Autodesk Inventor part; units mm, degrees
ref_plane "Work Plane1" through (0, 15, 0) normal (0, 1, 0) x (1, 0, 0)
ref_plane "Work Plane2" through (30.5, 0, 0) normal (1, 0, 0) x (0, 1, 0)
ref_plane "Work Plane6" through (0, 0, 2) normal (0, 0, 1) x (1, 0, 0)
sketch "Sketch1" plane through (0, 0, 0) normal (0, 1, 0) x (-1, 0, 0)
  circle A0 centre (0, 0) radius 26.5
  circle A1 centre (0, 0) radius 30.5
  dimension "d0" = 53
  dimension "d1" = 4
extrude "Extrusion1" add sketch "Sketch1" along normal blind 22
extrude "Extrusion2" add sketch "Sketch1" against normal blind 4 contours A0 | A1
ref_plane "Work Plane1" through (0, 15, 0) normal (0, 1, 0) x (1, 0, 0)
ref_plane "Work Plane2" through (30.5, 0, 0) normal (1, 0, 0) x (0, 1, 0)
sketch "Sketch3" plane through (30.5, 0, 0) normal (1, 0, 0) x (0, 1, 0)
  line L0 (14, -18.4883) -> (14, 18.4883)
  line L1 (16, 18.4883) -> (16, -18.4883)
  line L2 (16, 21.067) -> (16, 18.4883)
  line L3 (14, 18.4883) -> (14, 21.067)
  line L4 (16, 21.067) -> (16, -21.067)
  line L5 (16, 21.067) -> (16, 18.4883)
  line L6 (16, 18.4883) -> (16, -18.4883)
  line L7 (16, -18.4883) -> (16, -21.067)
  line L8 (14, -21.067) -> (14, -18.4883)
  line L9 (23, 32.2933) -> (-6, 32.2933)
  line L10 (-6, 32.2933) -> (-6, -38.454)
  line L11 (-6, -38.454) -> (23, -38.454)
  line L12 (23, -38.454) -> (23, 32.2933)
  line L13 (23, 24.5) -> (-6, 24.5)
  line L14 (23, -24.5) -> (-6.5731, -24.5)
  line L15 (-4, 30.5) -> (22, 30.5)
  line L16 (-4, -30.5) -> (22, -30.5)
  point P0 (0, 0)
  point P1 (-6, -24.5)
  dimension "d11" = 7
  dimension "d12" = 20
  dimension "d31" = 6
  dimension "d32" = 6
extrude "Extrusion4" cut sketch "Sketch3" against normal through all contours L12 L13 L10 L9 | L12 L11 L10 L14
sketch "Sketch4" plane through (0, 15, 0) normal (0, 1, 0) x (1, 0, 0)
  point P0 (0, 0)
ref_plane "Work Plane6" through (0, 0, 2) normal (0, 0, 1) x (1, 0, 0)
ref_plane "Work Plane5" through (0, 0, 30.5) normal (0, 0, 1) x (1, 0, 0)
sketch "Sketch6" plane through (0, 0, 2) normal (0, 0, 1) x (1, 0, 0)
  point P0 (0, 0)
sketch "Sketch7" plane through (0, 0, 2) normal (0, 0, 1) x (1, 0, 0)
  line L0 (-30.5, -4) -> (30.5, -4)
  line L1 (0, -4) -> (0, -71)
  circle A0 centre (0, -71) radius 57
  circle A1 centre (0, -71) radius 59.5
  circle A2 centre (0, -12.7932) radius 2.25
  circle A3 centre (-12.0008, -14) radius 2.25
  line L2 (4.6794, -4) -> (4.6794, -18.4597)
  line L3 (4.6794, -18.4597) -> (-15.0336, -19.4972)
  line L4 (-15.0336, -19.4972) -> (-17.1884, -4)
  point P0 (0, 0)
  dimension "d24" = 67
  dimension "d25" = 114
  dimension "d26" = 119
  dimension "d27" = 4.5
  dimension "d28" = 4.5
extrude "Extrusion6" add sketch "Sketch7" along normal mid plane 16 contours L0 L1 A2 A1 A3 L4 | L0 L2 A1 A2 L1 | A1 A3 A0 L4 | A0 A3 A2 L1 L3 L4 | L2 A0 A2 A1 | A2 A0 A3 A1 | L2 L3 L1 A2 A0
sketch "Sketch8" plane through (-18.1659, -4, 24.5) normal (0, 0, 1) x (1, 0, 0)
  line L0 (28.2654, 26) -> (36.3318, 26)
  line L1 (36.3318, 0) -> (0, 0)
  line L2 (36.3318, 26) -> (28.2654, 26)
  line L3 (28.2654, 26) -> (28.2654, 0)
  line L4 (28.2654, 0) -> (36.3318, 0)
  line L5 (36.3318, 0) -> (36.3318, 26)
  line L6 (28.2654, 4) -> (28.2654, 26)
  line L7 (0, 0) -> (0, 26)
  line L8 (36.3318, 0) -> (0, 0)
  line L9 (0, 0) -> (0, 4)
  line L10 (0, 4) -> (36.3318, 4)
  line L11 (36.3318, 4) -> (36.3318, 0)
  line L12 (8.0664, 26) -> (8.0664, 4)
  line L13 (0, 0) -> (8.0664, 0)
  line L14 (8.0664, 0) -> (8.0664, 26)
  line L15 (8.0664, 26) -> (0, 26)
  line L16 (0, 26) -> (0, 0)
  point P0 (18.1659, 4)
  dimension "d33" = 0
extrude "Extrusion7" add sketch "Sketch8" along normal blind 2
sketch "Sketch9" plane through (-18.1659, -4, 26.5) normal (0, 0, 1) x (1, 0, 0)
  line L0 (0, 0) -> (36.3318, 0)
  line L1 (8.0664, 26) -> (0, 26)
  line L2 (36.3318, 0) -> (0, 0)
  line L3 (0, 0) -> (0, 26)
  line L4 (0, 26) -> (36.3318, 26)
  line L5 (36.3318, 26) -> (36.3318, 0)
  line L6 (20.1659, 9) -> (16.1659, 9)
  line L7 (16.1659, 9) -> (16.1659, 26)
  line L8 (16.1659, 26) -> (20.1659, 26)
  line L9 (20.1659, 26) -> (20.1659, 9)
  line L10 (28.2654, 4) -> (8.0664, 4)
  point P0 (18.1659, 4)
  point P1 (18.1659, 4)
  point P2 (18.1659, 9)
  point P3 (18.1659, 4)
  dimension "d36" = 4
  dimension "d37" = 0
  dimension "d38" = 5
  dimension "d39" = 0
extrude "Extrusion8" add sketch "Sketch9" along normal blind 1 contours L3 L1 L4 L7 L6 L9 L5 L0
mirror "Mirror1" about plane through (0, 0, 0) normal (0, 0, 1) of "Extrusion8", "Extrusion7"
sketch "Sketch10" plane through (0, 22, 0) normal (0, 1, 0) x (1, 0, 0)
  circle A0 centre (0, 0) radius 28.75
  line L0 (10.0995, -24.5) -> (10.0995, -26.5)
  line L1 (10.0995, -26.5) -> (11.74, -26.5)
  line L2 (10.0995, -26.5) -> (11.74, -26.5) construction
  line L3 (11.74, -26.5) -> (-11.1496, -26.5)
  line L4 (27.6145, -8) -> (-27.6145, -8)
  point P0 (0, -8)
  point P1 (11.1496, -26.5)
  dimension "d42" = 57.5
  dimension "d43" = 0
  dimension "d44" = 8
extrude "Extrusion9" cut sketch "Sketch10" against normal up to surface (22 mm away) contours L4 A0 L1 L3
chamfer "Chamfer1" distance 2.25 angle 45 2 edges at (-25.2636, 11, 8) (25.2636, 11, 8)
mirror "Mirror2" about plane through (0, 0, 0) normal (0, 0, 1) of "Extrusion9"
chamfer "Chamfer2" distance 2.25 angle 45 2 edges at (-25.2636, 11, -8) (25.2636, 11, -8)
ref_plane "Work Plane7" through (4.6794, -4, 1) normal (0.1736, -0.9848, 0) x (0, 0, -1)
sketch "Sketch11" plane through (4.6794, -4, 1) normal (0.1736, -0.9848, 0) x (0, 0, -1)
  line L0 (-26.5, -22.4982) -> (-26.5, 13.2817)
  line L1 (28.5, -22.4982) -> (28.5, 13.2817)
  line L2 (7, -2.5109) -> (-9, -2.5109)
  line L3 (-9, 0) -> (7, 0)
  circle A0 centre (1, 0) radius 2.15
  point P0 (1, -3.9137)
  dimension "d54" = 4.3
  dimension "d55" = 27.5
extrude "Extrusion10" cut sketch "Sketch11" along normal through all both and the other way through all
ref_plane "Work Plane3" through (30.5, 0, 0) normal (1, 0, 0) x (0, 1, 0)
sketch "Sketch5" plane through (2, 0, 0) normal (1, 0, 0) x (0, 1, 0)
  line L0 (-4, 30.5) -> (-4, -30.5)
  line L1 (-4, 0) -> (-71, 0)
  circle A0 centre (-71, 0) radius 57
  circle A1 centre (-71, 0) radius 59.5
  circle A2 centre (-12.675, 0) radius 1.5
  circle A3 centre (-14.6323, 14.7617) radius 1.5
  line L2 (-4, -4.4838) -> (-16.1323, -4.4838)
  line L3 (-16.1323, -4.4838) -> (-19.3598, 18.592)
  line L4 (-19.3598, 18.592) -> (-4, 18.9349)
  point P0 (0, 0)
  dimension "d16" = 67
  dimension "d17" = 114
  dimension "d18" = 119
  dimension "d19" = 3
  dimension "d20" = 3
properties part number "BigLif2"
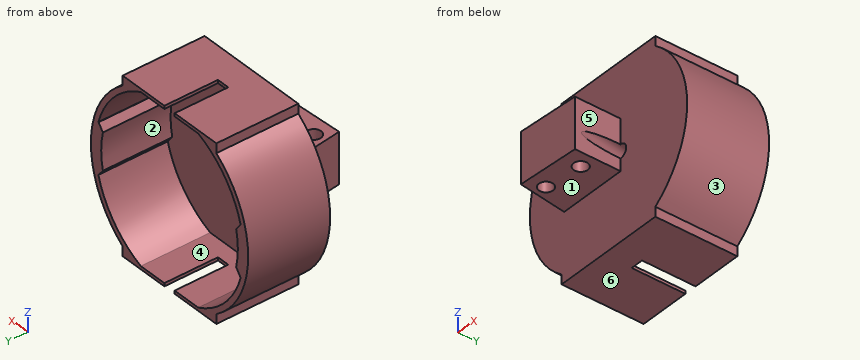
CAD build for the part. Positions are in the model's coordinates, mm. Face numbers are marked on the shaded views. A direction names the side the tool comes from. Round coordinates to 2 decimals unless told otherwise and drop trailing zeros. Order: outer loops, then holes, each group sorted by start corner. A loop starts at its lowest first (then second) coordinate and runs counter-clockwise, first axis right, second up. Notation, with made-up numbers: (-6.5, 36.25) - (-2.5, 36.25) arc R29 cw to (-2.5, 61.25) - close; hole circle Ø8 at (85.25, 45.5). An arc over 180 degrees is marked (long way). Answer in a Markdown table with one row per item. Add a question column.
(1) Drop flat-ended pins along their axis: pin 1 Ø6 at (x, y) = (0, -12.79) entering from -Z; pin 2 Ø1.1 at (y, z) = (16.5, 27) entering from +X; pin 3 Ø0.5 at (x, z) = (0, -27) entering from +Y; pin 4 Ø12 at (x, y) = (-23.5, -13) entering from -Z. Give the stop position or say it passes through.
(2) Band-saw the part on B-B on z = -21. List the corners of the cut face in (x, y).
(3) 3-axis set-ups, long thin cutter, end or side, ignore diameter. For the marked faces 4, 5 and 6: which of +Z, -Z, +X, -X, +Y, -Y reach the whole face in a straight line?
(4) Band-saw the part on D-D on y = -14. Count the separate pieces of the cut face and the enclosed holes in it, and give its area (3 significant figures).
(5) Band-saw the part on A-A on x = 0. List the corners of the cut face in (y, z), and give its area (3 significant figures).
(6) Probe L1, parallel to Z at x = 8, y = 15; L2, parallel to X at y = -14, z = 4; L3, parallel to Y at x = 11, z = 17. List the from-to ranges inside material, lowest first. Write a range as [from, to].
(7) Band-saw the part on C-C on x = 22. List the corners of the cut face in (y, z), and give its area (3 significant figures).
(8) Mould opens along X. For the marked faces 1, 2 and 3 say: +X half, -X half, draft (parallel to the pull), parting line (faces both ways), or undercut.
Data:
| question | item | result |
|---|---|---|
| 1 | pin 1 | stops at z = -6 |
| 1 | pin 2 | stops at x = 18.17 |
| 1 | pin 3 | stops at y = 5 |
| 1 | pin 4 | passes through |
| 2 | outline | (-22.12, -4) - (22.12, -4) - (22.12, 22) - (19.64, 22) - (19.64, 0) - (-19.64, 0) - (-19.64, 22) - (-22.12, 22) - close |
| 3 | face 4 | +Y |
| 3 | face 5 | +Z, -Z, +X, -Y |
| 3 | face 6 | -Z, +X, -X, +Y, -Y |
| 4 | separate pieces | 3 |
| 4 | enclosed holes | 0 |
| 4 | area | 194 mm^2 |
| 5 | outline | (-18.71, -6) - (-15.04, -6) - (-15.04, 10) - (-18.71, 10) - close; (-10.54, -6) - (-4, -6) - (-4, -27.5) - (5, -27.5) - (5, -26.5) - (0, -26.5) - (0, 26.5) - (5, 26.5) - (5, 27.5) - (-4, 27.5) - (-4, 10) - (-10.54, 10) - close |
| 5 | area | 393 mm^2 |
| 6 | L1 | z = [-27.5, -26.5], [26.5, 27.5] |
| 6 | L2 | x = [-15.8, -14.25], [-9.75, -1.9], [1.9, 4.68] |
| 6 | L3 | y = [-4, 0] |
| 7 | outline | (-4, -21.12) - (22, -21.12) - (22, -18.51) - (0, -18.51) - (0, 18.51) - (22, 18.51) - (22, 21.12) - (-4, 21.12) - close |
| 7 | area | 284 mm^2 |
| 8 | face 1 | draft |
| 8 | face 2 | undercut |
| 8 | face 3 | +X half |
